Autodesk Inventor part; units mm, degrees
ref_plane "YZ Plane" through (0, 0, 0) normal (1, 0, 0) x (0, 1, 0)
ref_plane "XZ Plane" through (0, 0, 0) normal (0, 1, 0) x (-1, 0, 0)
ref_plane "XY Plane" through (0, 0, 0) normal (0, 0, 1) x (1, 0, 0)
sketch "スケッチ1" plane through (0, 0, 0) normal (0, 1, 0) x (-1, 0, 0)
  circle A0 centre (0, 0) radius 3.1754 construction
  line L0 (3.1754, 0) -> (1.5877, 2.75)
  line L1 (1.5877, 2.75) -> (-1.5877, 2.75)
  line L2 (-1.5877, 2.75) -> (-3.1754, 0)
  line L3 (-3.1754, 0) -> (-1.5877, -2.75)
  line L4 (-1.5877, -2.75) -> (1.5877, -2.75)
  line L5 (1.5877, -2.75) -> (3.1754, 0)
  dimension "d0" = 5.5
extrude "押し出し1" add sketch "スケッチ1" along normal blind 2.4
sketch "スケッチ2" plane through (0, 2.4, 0) normal (0, 1, 0) x (1, 0, 0)
  point P0 (0, 0)
  point P1 (0, 0)
hole "穴1" at (0, 2.4, 0) direction (0, -1, 0) diameter 2.459 end through all
sketch "スケッチ3" plane through (0, 0, 0) normal (1, 0, 0) x (0, 1, 0)
  arc A0 (1.7511, -3.75) -> (2.4, -2.75) centre (-2.9327, 0) ccw
  line L0 (0, -2.75) -> (2.4, -2.75) construction
  line L1 (2.4, -3.75) -> (1.7511, -3.75)
  line L2 (2.4, 1.2295) -> (2.4, -1.2295) construction
  line L3 (2.4, -2.75) -> (2.4, -3.75)
  line L4 (-4.0042, 0) -> (3.4964, 0)
  point P0 (0, 0)
  point P1 (2.4, 0)
  dimension "d10" = 2.75
  dimension "d11" = 6
  dimension "d12" = 1
revolve "回転1" cut sketch "スケッチ3" angle 360 about axis through (0, -10, 0) along (0, 1, 0)
properties part number "M3-HexaNut-type2"
Here's how the part is built. I have some questions about the finished solid (model axes, mm). Give positions to 0.01 mm unless a question says otherwise; leave off trailing zeros. Order: outer loops, then holes, each group sorted by start corner. A loop starts at its lowest first (then second) coordinate and runs counter-clockwise, first axis right, second up. Notation, with made-up numbers: M 37,-18 L 55,-18 A4 ccw 55,-14 Z; hole C -6,59.5 d1. An arc over 180 degrees is marked long. Use a Markdown table: item, result. Add a question column.
1. I need wall thicknesses on probe 1 along Z at (x, y) = (0, 1.25); probe 2 along Z at (x, y) = (0.5, 0.35); probe 3 along Y at (x, z) = (-1.25, 2.5). Which ranges of each line are inside material? Lowest first, please. Write a range as from..to.
2. For pin 1 Ø1 at (y, z) = (1.5, -1.5) entering from +X, with a flat end and sliding along its axis, tell me the tip position at first contact or that it passes through.
3. If we mould it in two halves opening along X, with no side actions, what happens to faces 1 (the flat face through (-2.39, 1.18, 1.36)), 2 (the flat face through (-1.4, 0, 0)), 3 (the flat face through (2.37, 1.183, 1.394)), 4 (the cylindrical face through (0.748, 1.183, -0.976))? For each: +X half, -X half, draft (parallel to the pull), parting line (faces both ways), or undercut.
4. Suppose I cut it at A-A (y = 1.6). List the corners of the cut face in (x, z) for me.
Results list:
| question | item | result |
|---|---|---|
| 1 | probe 1 | z = -2.75..-1.23, 1.23..2.75 |
| 1 | probe 2 | z = -2.75..-1.12, 1.12..2.75 |
| 1 | probe 3 | y = 0..2.38 |
| 2 | pin 1 | stops at x = 2.6 |
| 3 | face 1 | -X half |
| 3 | face 2 | draft |
| 3 | face 3 | +X half |
| 3 | face 4 | undercut |
| 4 | outline | M -3.18,0 L -1.59,-2.75 L 1.59,-2.75 L 3.18,0 L 1.59,2.75 L -1.59,2.75 Z; hole C 0,0 d2.46 |
